```python
from build123d import *


with BuildPart() as f2:
    # F2: sweep along a path in F0
    with BuildLine(Plane.XY) as f2_path:
        Line((-373.5, 286), (-373.5, -286))
        Line((-373.5, -286), (373.5, -286))
        Line((373.5, -286), (373.5, 286))
        Line((373.5, 286), (-373.5, 286))
    # F1 (on Front) → F2 (sweep)
    with BuildSketch(Plane.XZ):
        Polygon((-372.3, 12), (-373.5, 12), (-373.5, 0), (-361.5, 0), (-361.5, 1.2), (-372.3, 1.2), align=None)
    sweep(path=f2_path.line, transition=Transition.RIGHT)


solid = f2.part
```
Read the model definition and answer for the solid it produces. Units are mm, in the model's axes. Round coordinates to 2 decimals unless told otherwise and drop trailing zeros. Write each loop counter-clockwise with the first axis right and the second up, starting at its lowest first coordinate (ties: lowest second). Pieces come first, ordered by that corner, then holes. Notation, with made-up numbers: (31, 70) -> (69, 70) arc R25 cw to (69, 100) -> close; hole circle Ø11 at (7, 30.5). An arc over 180 degrees is marked (long way). Answer in a Markdown table with one row per item. Add a question column.
1) Determine the mould class of faces 1 (the face through (-2, -277, 0)), 2 (the face through (2, -276, 1.2)) for opening direction Y: pulls with the +Y half, pulls with the -Y half, needs draft (parallel to the pull), parting line crosses it, or undercut.
2) Find section B-B, the plane z = 5.5. Determine the outline of the cut face in (x, y).
3) Find section C-C, the plane x = -325. Determine the outline of the cut face in (y, z), and give its area (3 significant figures).
4) Find section A-A, the plane y = 54. Determine the outline of the cut face in (x, z).
5) Consider line 1 (X direction, y = 206.5, z = 6.5); line 2 (Y direction, x = 150, z = 8.5). Determine where each line is inside the solid, lowest interval first.
Findings below:
| question | item | result |
|---|---|---|
| 1 | face 1 | needs draft |
| 1 | face 2 | undercut |
| 2 | outline | (-373.5, -286) -> (373.5, -286) -> (373.5, 286) -> (-373.5, 286) -> close; hole (-372.3, -284.8) -> (372.3, -284.8) -> (372.3, 284.8) -> (-372.3, 284.8) -> close |
| 3 | outline | (-286, 0) -> (-274, 0) -> (-274, 1.2) -> (-284.8, 1.2) -> (-284.8, 12) -> (-286, 12) -> close; (274, 0) -> (286, 0) -> (286, 12) -> (284.8, 12) -> (284.8, 1.2) -> (274, 1.2) -> close |
| 3 | area | 54.7 mm² |
| 4 | outline | (-373.5, 0) -> (-361.5, 0) -> (-361.5, 1.2) -> (-372.3, 1.2) -> (-372.3, 12) -> (-373.5, 12) -> close; (361.5, 0) -> (373.5, 0) -> (373.5, 12) -> (372.3, 12) -> (372.3, 1.2) -> (361.5, 1.2) -> close |
| 5 | line 1 | -373.5 to -372.3, 372.3 to 373.5 |
| 5 | line 2 | -286 to -284.8, 284.8 to 286 |
